The model under review builds one solid part; all positions refer to its coordinate system, in mm. Coordinates: 2 decimals unless noted, no trailing zeros. Order: outer loops, then holes, each group sorted by start corner. A loop starts at its lowest first (then second) coordinate and runs counter-clockwise, first axis right, second up. Notation, with made-up numbers: M 75.25,40.25 L 116.25,40.25 A27 cw 116.25,69.25 Z; hole C 63,69.5 d4. An arc over 180 degrees is marked long. Answer in a Markdown table with one row per item.
from build123d import *

# Parameters (mm, degrees)
SKETCH002_R              = 3.2
PAD001_DEPTH             = 200
FILLET_R                 = 1
FILLET001_R              = 1
CLONE003_PLACEMENT_ANGLE = 90


with BuildPart() as part:
    # Sketch002 (on DatumPlane) → Pad001 (new body)
    with BuildSketch(Plane(origin=(0, -40, 70), x_dir=(1, 0, 0), z_dir=(0, -1, 0))):
        with Locations((20, -50)):
            Circle(SKETCH002_R)
    extrude(amount=-PAD001_DEPTH)

    # Fillet
    fillet_edges = [part.edges().sort_by_distance(p)[0] for p in [
        (16.8, -40, 20),
    ]]
    fillet(fillet_edges, radius=FILLET_R)

    # Fillet001
    fillet001_edges = [part.edges().sort_by_distance(p)[0] for p in [
        (16.8, 160, 20),
    ]]
    fillet(fillet001_edges, radius=FILLET001_R)


with BuildPart() as part_1:
    # Clone003 placement: moved
    add(part.part.rotate(Axis((0, 0, 0), (0, -1, 0)), CLONE003_PLACEMENT_ANGLE))


solid = part_1.part
(1) To check wall thickness, follow line 1 (Y direction, x = -19.5, z = 22.25); line 2 (X direction, y = 109, z = 20.25); line 3 (X direction, y = 19, z = 17.5). State the ranges of each line that lie inside material, in increasing order. Write a range as [from, to].
Report:
| item | result |
|---|---|
| line 1 | [-39.99, 159.99] |
| line 2 | [-23.19, -16.81] |
| line 3 | [-22, -18] |
(2) Take a section at A-A (y = 5.5). Write out the cut boundary in (x, z), then the cut area to 3 significant figures.
Report:
| item | result |
|---|---|
| outline | C -20,20 d6.4 |
| area | 32.2 mm^2 |
(3) Insertion check: P1, Ø1, axis at y = 135.5, z = 18.5, coming from the +X side; P2, Ø2, axis at y = 92.5, z = 18.5, coming from the +X side; P3, Ø3, axis at x = -17.5, y = 35.5, coming from the +Z side. Each pin has a flat end and moves straight along its axis. Give the tip position at first contact, or say it passes through.
Report:
| item | result |
|---|---|
| P1 | x = -16.96 |
| P2 | x = -16.84 |
| P3 | z = 23.04 |
